Input: part model. Units: mm. Frame: model coordinates. Face numbers are marked on the shaded views. A direction names the side the tool comes from. Give positions to 0.01 mm unless a question says otherwise; leave off trailing zeros. Write each loop counter-clockwise with the first axis right and the second up, starting at its lowest first coordinate (ties: lowest second). Pieces come first, ordered by that corner, then holes.
```python
from build123d import *

# Parameters (mm, degrees)
BOSS_EXTRUDE1_DEPTH = 19
CUT_EXTRUDE1_DEPTH  = 28.092434368
CUT_EXTRUDE2_DEPTH  = 1
SKETCH4_W           = 6
SKETCH4_H           = 16
CUT_EXTRUDE3_DEPTH  = 5


with BuildPart() as part:
    # Sketch1 → Boss-Extrude1 (new body)
    with BuildSketch(Plane.XY):
        Polygon((0, 0), (18, 0), (18, 4), (9, 4), (8.5, 4), (8.5, 4.5), (9, 4.5), (9, 7), (0, 7), align=None)
    extrude(amount=BOSS_EXTRUDE1_DEPTH)

    # Sketch2 → Cut-Extrude1 (cut, through all)
    with BuildSketch(Plane(origin=(0, 7, 0), x_dir=(1, 0, 0), z_dir=(0, 1, 0))):
        with BuildLine():
            Line((13.5, -2.4), (18, -2.4))
            Line((18, -2.4), (18, -6.6))
            Line((18, -6.6), (13.5, -6.6))
            ThreePointArc((13.5, -6.6), (11.4, -4.5), (13.5, -2.4))
        make_face()
        with BuildLine():
            Line((13.5, -12.4), (18, -12.4))
            Line((18, -12.4), (18, -16.6))
            Line((18, -16.6), (13.5, -16.6))
            ThreePointArc((13.5, -16.6), (11.4, -14.5), (13.5, -12.4))
        make_face()
    extrude(amount=-CUT_EXTRUDE1_DEPTH, mode=Mode.SUBTRACT)

    # Sketch3 → Cut-Extrude2 (cut)
    # profile 1 of 3: a face of its own
    with BuildSketch(Plane(origin=(0, 7, 0), x_dir=(1, 0, 0), z_dir=(0, 1, 0))):
        Polygon((6.307692308, -7.314182692), (6.307692308, -8.1), (3.561538462, -8.1), (3.561538462, -8.476923077), (2.861538462, -8.476923077), (2.861538462, -8.1), (2, -8.1), (2, -7.346153846), (2.861538462, -7.346153846), (2.861538462, -5.569230769), (3.624639423, -5.569230769), align=None)
        Polygon((3.561538462, -7.346153846), (4.990985577, -7.346153846), (3.561538462, -6.416466346), align=None, mode=Mode.SUBTRACT)
    # profile 2 of 3: a face of its own
    with BuildSketch(Plane(origin=(0, 7, 0), x_dir=(1, 0, 0), z_dir=(0, 1, 0))):
        with BuildLine():
            add(Edge.make_bspline(
                [(2.861538462, -9.526923077), (2.85988287, -9.557362204), (2.856623295, -9.617291589), (2.831853959, -9.703995704), (2.788312606, -9.782702644), (2.730502257, -9.85257974), (2.661701966, -9.911911527), (2.582376507, -9.953401025), (2.496427686, -9.98023852), (2.436302157, -9.983133621), (2.405528846, -9.984615385)],
                knots=[0, 0, 0, 0, 1.016476041, 2.001265769, 2.982571086, 4.001334304, 5.018889842, 5.99575474, 6.974191785, 8, 8, 8, 8], degree=3))
            add(Edge.make_bspline(
                [(2.405528846, -9.984615385), (2.374750787, -9.983143332), (2.31461598, -9.980267206), (2.228495667, -9.95321757), (2.148526587, -9.911977622), (2.078984136, -9.852574786), (2.020088959, -9.78299344), (1.976959039, -9.703815063), (1.950796284, -9.617456418), (1.947716214, -9.557391196), (1.946153846, -9.526923077)],
                knots=[0, 0, 0, 0, 1.022731703, 1.998234309, 2.980426153, 4.002090265, 5.023754376, 6.00211665, 6.986572482, 8, 8, 8, 8], degree=3))
            add(Edge.make_bspline(
                [(1.946153846, -9.526923077), (1.947729022, -9.496462175), (1.950834344, -9.436411182), (1.976740674, -9.350186567), (2.020380314, -9.271588463), (2.078913136, -9.202024595), (2.14877397, -9.142885964), (2.228244922, -9.100439216), (2.314648555, -9.073639214), (2.374761815, -9.070723224), (2.405528846, -9.069230769)],
                knots=[0, 0, 0, 0, 1.013910294, 1.9988351, 2.969460266, 3.991611077, 5.013761889, 6.000813773, 6.976781088, 8, 8, 8, 8], degree=3))
            add(Edge.make_bspline(
                [(2.405528846, -9.069230769), (2.436290937, -9.070733066), (2.496394544, -9.073668284), (2.582630141, -9.100255237), (2.661453239, -9.142949764), (2.730573405, -9.202019856), (2.788023525, -9.271877769), (2.832069332, -9.350006935), (2.856584954, -9.436576095), (2.859869955, -9.496491201), (2.861538462, -9.526923077)],
                knots=[0, 0, 0, 0, 1.02629359, 2.005193596, 2.986963232, 4.00500024, 5.0242455, 5.997787305, 6.983042999, 8, 8, 8, 8], degree=3))
        make_face()
    # profile 3 of 3: a face of its own
    with BuildSketch(Plane(origin=(0, 7, 0), x_dir=(1, 0, 0), z_dir=(0, 1, 0))):
        with BuildLine():
            add(Edge.make_bspline(
                [(6.307692308, -11.937379808), (6.307150683, -11.973869128), (6.306085705, -12.045616881), (6.29454866, -12.151287171), (6.277124504, -12.25307935), (6.252805809, -12.351380113), (6.220685788, -12.445523764), (6.18190987, -12.536269402), (6.135550949, -12.622853881), (6.082281439, -12.705477488), (6.02270567, -12.784525027), (5.953841518, -12.857366744), (5.878739381, -12.926822083), (5.796159568, -12.991739367), (5.705539209, -13.051391781), (5.608078808, -13.106892863), (5.502860985, -13.157526901), (5.389778503, -13.20396373), (5.267117399, -13.245505969), (5.133456997, -13.280398151), (4.988893108, -13.310732399), (4.832672601, -13.334621473), (4.665163984, -13.354174114), (4.486053808, -13.366949594), (4.295843307, -13.375837098), (4.16535578, -13.376554506), (4.098317308, -13.376923077)],
                knots=[0, 0, 0, 0, 0.879087513, 1.728520926, 2.558587148, 3.366762743, 4.166157112, 4.95337177, 5.74258602, 6.530032775, 7.320866164, 8.124307838, 8.942260106, 9.784645725, 10.652593514, 11.554662219, 12.485739241, 13.464770064, 14.499274465, 15.604285219, 16.792026686, 18.057713884, 19.411711354, 20.855437135, 22.384468668, 24, 24, 24, 24], degree=3))
            add(Edge.make_bspline(
                [(4.098317308, -13.376923077), (4.030440525, -13.37652196), (3.898557155, -13.375742597), (3.70660119, -13.367345458), (3.526210383, -13.3528853), (3.357403645, -13.334247649), (3.200269274, -13.308720394), (3.054403265, -13.278820445), (2.919848806, -13.243303124), (2.79694166, -13.200378221), (2.68359105, -13.154337682), (2.578944999, -13.103208582), (2.481123496, -13.050067474), (2.391489769, -12.991693005), (2.309846766, -12.929325786), (2.235444428, -12.863944923), (2.169307235, -12.794157234), (2.110069404, -12.7210064), (2.058216793, -12.642714885), (2.01366831, -12.55962707), (1.976853175, -12.471182306), (1.9451208, -12.378667246), (1.922290893, -12.280436063), (1.90419103, -12.178005479), (1.894184694, -12.070231506), (1.892943628, -11.99685416), (1.892307692, -11.959254808)],
                knots=[0, 0, 0, 0, 1.643682949, 3.193646483, 4.651618242, 6.025629174, 7.305184366, 8.505292942, 9.630500342, 10.672179876, 11.655924581, 12.591484594, 13.491256898, 14.350247848, 15.17884557, 15.977481787, 16.746098769, 17.504475725, 18.254166354, 19.016819136, 19.783753977, 20.571954997, 21.382401421, 22.223156612, 23.089526058, 24, 24, 24, 24], degree=3))
            add(Edge.make_bspline(
                [(1.892307692, -11.959254808), (1.892958632, -11.921657209), (1.894233814, -11.848004067), (1.904086281, -11.739928272), (1.922520224, -11.636723558), (1.944975925, -11.537578193), (1.977024282, -11.443362893), (2.014430371, -11.353389364), (2.059233294, -11.268105532), (2.110855853, -11.187457673), (2.170065111, -11.11173783), (2.236213665, -11.03976485), (2.309137681, -10.971699163), (2.389652904, -10.908575843), (2.476684941, -10.84936136), (2.571227482, -10.794672603), (2.673143257, -10.744544816), (2.782572889, -10.697400516), (2.901878097, -10.656467963), (3.032100284, -10.619915704), (3.174468576, -10.590475047), (3.328448015, -10.564687625), (3.494578206, -10.547373), (3.672092814, -10.532564683), (3.861539617, -10.524279313), (3.991739434, -10.523485583), (4.058774038, -10.523076923)],
                knots=[0, 0, 0, 0, 0.917197984, 1.796777363, 2.643741708, 3.473481078, 4.273990801, 5.068160217, 5.848535553, 6.620952589, 7.401027954, 8.190319769, 9.003592045, 9.831693788, 10.683727512, 11.569696396, 12.49373307, 13.453184301, 14.474457586, 15.568383184, 16.750575061, 18.019320986, 19.375517054, 20.823796471, 22.364701649, 24, 24, 24, 24], degree=3))
            add(Edge.make_bspline(
                [(4.058774038, -10.523076923), (4.151913091, -10.523808273), (4.331626093, -10.525219423), (4.591295751, -10.542644047), (4.83113749, -10.569002763), (5.051441104, -10.605085819), (5.251775391, -10.653685764), (5.432082806, -10.713328421), (5.594148159, -10.781764373), (5.690172203, -10.839987872), (5.736418269, -10.868028846)],
                knots=[0, 0, 0, 0, 1.288526675, 2.486228817, 3.599112392, 4.626206381, 5.5730174, 6.447949553, 7.252518174, 8, 8, 8, 8], degree=3))
            add(Edge.make_bspline(
                [(5.736418269, -10.868028846), (5.781849131, -10.900640072), (5.870675418, -10.964401446), (5.987287729, -11.07588999), (6.087020287, -11.195669914), (6.167616056, -11.326201431), (6.231173886, -11.46542013), (6.276064066, -11.614521274), (6.302219176, -11.772954258), (6.305840687, -11.881752831), (6.307692308, -11.937379808)],
                knots=[0, 0, 0, 0, 1.058512271, 2.069600068, 3.047294572, 4.004278952, 4.967380941, 5.939006123, 6.946246673, 8, 8, 8, 8], degree=3))
        make_face()
        with BuildLine():
            add(Edge.make_bspline(
                [(5.553846154, -11.955889423), (5.552270668, -11.922908887), (5.54918188, -11.858249528), (5.523401693, -11.764568479), (5.48271655, -11.676626924), (5.434760512, -11.609308285), (5.387973655, -11.559148094), (5.34693293, -11.522793846), (5.298932536, -11.490234906), (5.246047261, -11.458820008), (5.186821663, -11.430869169), (5.12274956, -11.403076295), (5.051691887, -11.380433104), (4.974987834, -11.358133021), (4.89047493, -11.338636996), (4.797488532, -11.322180048), (4.695329433, -11.307988824), (4.584245274, -11.296006011), (4.463793783, -11.288387596), (4.3342554, -11.281014932), (4.195362046, -11.278331006), (4.099719168, -11.277402337), (4.050360577, -11.276923077)],
                knots=[0, 0, 0, 0, 1.076821401, 2.111141558, 3.153197101, 4.23200803, 4.796476379, 5.394298193, 6.020090776, 6.690078086, 7.403703365, 8.159894791, 8.971856079, 9.83973388, 10.771758647, 11.806038152, 12.926526118, 14.143777411, 15.458313878, 16.872423957, 18.385946227, 20, 20, 20, 20], degree=3))
            add(Edge.make_bspline(
                [(4.050360577, -11.276923077), (3.986412475, -11.277690687), (3.863787247, -11.279162637), (3.687454343, -11.286901656), (3.526954651, -11.302324436), (3.381298609, -11.321757427), (3.251038899, -11.348230248), (3.136135085, -11.381192718), (3.035736471, -11.41774611), (2.951319527, -11.463577141), (2.879125714, -11.512681076), (2.816674456, -11.565091786), (2.764651799, -11.621723368), (2.720485601, -11.680883073), (2.687689615, -11.744764797), (2.663780285, -11.812058623), (2.649202201, -11.882913935), (2.647175838, -11.931423642), (2.646153846, -11.955889423)],
                knots=[0, 0, 0, 0, 1.772047989, 3.398033405, 4.888860297, 6.238411839, 7.468309579, 8.567754056, 9.549141588, 10.421774021, 11.221426488, 11.965694757, 12.675067502, 13.348095901, 14.005005053, 14.656328889, 15.322321954, 16, 16, 16, 16], degree=3))
            add(Edge.make_bspline(
                [(2.646153846, -11.955889423), (2.64685234, -11.979516527), (2.648219904, -12.025775459), (2.662257763, -12.093231342), (2.685080272, -12.157022417), (2.717364314, -12.216956081), (2.758418413, -12.273246707), (2.808422978, -12.325619182), (2.867876439, -12.373678523), (2.911999699, -12.401678113), (2.934735577, -12.416105769)],
                knots=[0, 0, 0, 0, 0.992283464, 1.942767638, 2.88273346, 3.832339453, 4.79467288, 5.803907806, 6.868395428, 8, 8, 8, 8], degree=3))
            add(Edge.make_bspline(
                [(2.934735577, -12.416105769), (2.965802388, -12.43309715), (3.030946973, -12.468726699), (3.140897888, -12.509852713), (3.264748166, -12.544936354), (3.403499208, -12.573060354), (3.556594281, -12.59533645), (3.724147171, -12.61236653), (3.906398045, -12.62101668), (4.032684545, -12.622372359), (4.098317308, -12.623076923)],
                knots=[0, 0, 0, 0, 0.710996797, 1.490902623, 2.352723643, 3.296875318, 4.334065587, 5.461510359, 6.680713396, 8, 8, 8, 8], degree=3))
            add(Edge.make_bspline(
                [(4.098317308, -12.623076923), (4.164517758, -12.622799909), (4.291942324, -12.622266703), (4.474875271, -12.612483906), (4.641954183, -12.598860635), (4.79280593, -12.578933654), (4.927797071, -12.55329418), (5.046917647, -12.521692777), (5.150406, -12.484439109), (5.238147698, -12.440254292), (5.312742503, -12.391337042), (5.37665067, -12.339343271), (5.431670617, -12.284183068), (5.476266621, -12.225262109), (5.511810773, -12.162973601), (5.536033359, -12.096981471), (5.55093428, -12.027505248), (5.552862428, -11.980083575), (5.553846154, -11.955889423)],
                knots=[0, 0, 0, 0, 1.793903324, 3.452957663, 4.963427329, 6.336122014, 7.574844885, 8.684777121, 9.673127442, 10.55010789, 11.340650774, 12.086136756, 12.779466299, 13.446812155, 14.083183996, 14.715685896, 15.34475337, 16, 16, 16, 16], degree=3))
        make_face(mode=Mode.SUBTRACT)
    extrude(amount=-CUT_EXTRUDE2_DEPTH, mode=Mode.SUBTRACT)

    # Sketch4 → Cut-Extrude3 (cut)
    with BuildSketch(Plane.XZ):
        with Locations((4.5, 9.5)):
            Rectangle(SKETCH4_W, SKETCH4_H)
    extrude(amount=-CUT_EXTRUDE3_DEPTH, mode=Mode.SUBTRACT)


solid = part.part
```
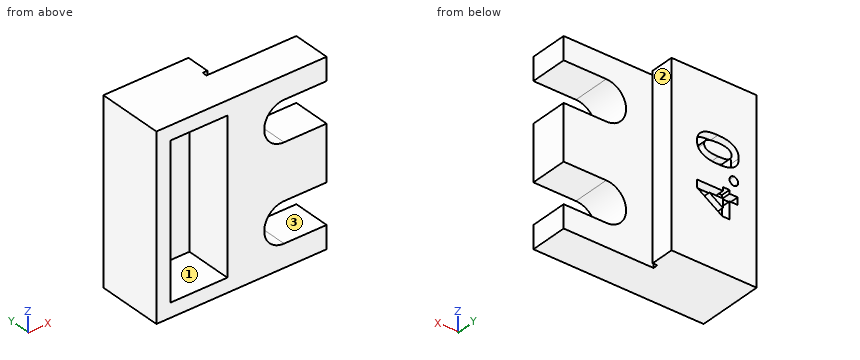
Item 1: Pin query (flat end, axial travel): pin 1 (1 mm diameter, centred on y = 5.5, z = 12, fed in from -X); pin 2 (0.5 mm diameter, centred on y = 6.5, z = 6.5, fed in from +X); pin 3 (2 mm diameter, centred on y = 1.5, z = 4.5, fed in from +X). Return the tip coordinate at first contact, or that it passes through.
Item 2: Section B-B (y = 3.75). Return loops of the section in (x, z), and give its area (3 significant figures).
Item 3: Set-up query: the marked faces 1, 2 and 3. Return all of +Z, -Z, +X, -X, +Y, -Y with unobstructed straight access to the full face (end or side cutting, diameter ignored); none if empty.
Item 4: Ray query, line 1 (Z direction, x = 17, y = 2); line 2 (X direction, y = 2, z = 14.5); line 3 (X direction, y = 3, z = 1.75). Return the intervals inside material, ascending.
Item 5: Section A-A (x = 14.5). Return loops of the section in (y, z).
Item 6: Section D-D (y = 5.25). Return loops of the section in (x, z), and give its area (3 significant figures).
Item 7: Section C-C (z = 4.5). Return loops of the section in (x, y), and give its area (4 significant figures).
Solved:
1. pin 1: stops at x = 0
1. pin 2: stops at x = 9
1. pin 3: stops at x = 11.65
2. outline: (0, 0) - (18, 0) - (18, 2.4) - (13.5, 2.4) arc R2.1 cw to (13.5, 6.6) - (18, 6.6) - (18, 12.4) - (13.5, 12.4) arc R2.1 cw to (13.5, 16.6) - (18, 16.6) - (18, 19) - (0, 19) - close; hole (1.5, 1.5) - (7.5, 1.5) - (7.5, 17.5) - (1.5, 17.5) - close
2. area: 194 mm2
3. face 1: -Y
3. face 2: +Z, -Z, +X, +Y
3. face 3: +X, +Y, -Y
4. line 1: z = 0 to 2.4, 6.6 to 12.4, 16.6 to 19
4. line 2: x = 0 to 1.5, 7.5 to 11.4
4. line 3: x = 0 to 1.5, 7.5 to 18
5. outline: (0, 0) - (4, 0) - (4, 2.4) - (0, 2.4) - close; (0, 6.6) - (4, 6.6) - (4, 12.4) - (0, 12.4) - close; (0, 16.6) - (4, 16.6) - (4, 19) - (0, 19) - close
6. outline: (0, 0) - (9, 0) - (9, 19) - (0, 19) - close
6. area: 171 mm2
7. outline: (0, 0) - (1.5, 0) - (1.5, 5) - (7.5, 5) - (7.5, 0) - (11.4, 0) - (11.4, 4) - (8.5, 4) - (8.5, 4.5) - (9, 4.5) - (9, 7) - (0, 7) - close
7. area: 42.35 mm2
